The model under review builds one solid part; all positions refer to its coordinate system, in mm. Face numbers are marked on the shaded views. A direction names the side the tool comes from. Coordinates: 2 decimals unless noted, no trailing zeros. Write each loop counter-clockwise with the first axis right and the second up, starting at its lowest first coordinate (ties: lowest second). Pieces come first, ordered by that corner, then holes.
```python
from build123d import *

# Parameters (mm, degrees)
SKETCH1_R               = 20
BOSS_EXTRUDE1_DEPTH     = 60
CUT_EXTRUDE1_DEPTH      = 67.332495807
CUT_EXTRUDE1_DEPTH_BACK = 67.332495807
SKETCH2_R               = 10
FILLET1_R               = 3
SKETCH22_R              = 17
BOSS_EXTRUDE4_DEPTH     = 100
CUT_EXTRUDE4_DEPTH      = 100
CUT_EXTRUDE4_DEPTH_BACK = 100
SKETCH19_R              = 10
CUT_EXTRUDE5_START      = -80
CUT_EXTRUDE5_DEPTH      = 80


with BuildPart() as part:
    # Sketch1 → Boss-Extrude1 (new body)
    with BuildSketch(Plane.XY):
        Circle(SKETCH1_R)
    extrude(amount=BOSS_EXTRUDE1_DEPTH)

    # Sketch2 → Cut-Extrude1 (cut, two sides: drawn at the far end of the back side and taken through both)
    with BuildSketch(Plane(origin=(0, 0, 0), x_dir=(1, 0, 0), z_dir=(0, 1, 0)).offset(-CUT_EXTRUDE1_DEPTH_BACK)):
        with Locations(Location((0, -30, 0), (0, 0, 270))):
            Circle(SKETCH2_R)
    extrude(amount=CUT_EXTRUDE1_DEPTH + CUT_EXTRUDE1_DEPTH_BACK, mode=Mode.SUBTRACT)

    # Fillet1
    fillet1_edges = [part.edges().sort_by_distance(p)[0] for p in [
        (-20, 0, 0),
        (-20, 0, 60),
    ]]
    fillet(fillet1_edges, radius=FILLET1_R)

    # Sketch22 → Boss-Extrude4 (add)
    with BuildSketch(Plane.XY.offset(60)):
        Circle(SKETCH22_R)
    extrude(amount=BOSS_EXTRUDE4_DEPTH)

    # Sketch19 → Cut-Extrude4 (cut, two sides: drawn at the far end of the back side and taken through both)
    with BuildSketch(Plane(origin=(0, 0, 0), x_dir=(1, 0, 0), z_dir=(0, 1, 0)).offset(-CUT_EXTRUDE4_DEPTH_BACK)):
        with Locations(Location((0, -120, 0), (0, 0, 90))):
            Circle(SKETCH19_R)
    extrude(amount=CUT_EXTRUDE4_DEPTH + CUT_EXTRUDE4_DEPTH_BACK, mode=Mode.SUBTRACT)

    # Sketch23 → Cut-Extrude5 (cut)
    with BuildSketch(Plane.XY.offset(160).offset(CUT_EXTRUDE5_START)):
        with BuildLine():
            ThreePointArc((12.56265543, 11.453370183), (0, 17), (-12.56265543, 11.453370183))
            Line((-12.56265543, 11.453370183), (12.56265543, 11.453370183))
        make_face()
        with BuildLine():
            Line((-12.56265543, -11.453370183), (-12.56265543, 11.453370183))
            ThreePointArc((-12.56265543, 11.453370183), (-17, 0), (-12.56265543, -11.453370183))
        make_face()
        with BuildLine():
            Line((12.56265543, -11.453370183), (-12.56265543, -11.453370183))
            ThreePointArc((-12.56265543, -11.453370183), (0, -17), (12.56265543, -11.453370183))
        make_face()
        with BuildLine():
            ThreePointArc((17, 0), (15.851894876, 6.141451689), (12.56265543, 11.453370183))
            Line((12.56265543, 11.453370183), (12.56265543, -11.453370183))
            ThreePointArc((12.56265543, -11.453370183), (15.851894876, -6.141451689), (17, 0))
        make_face()
    extrude(amount=CUT_EXTRUDE5_DEPTH, mode=Mode.SUBTRACT)


solid = part.part
```
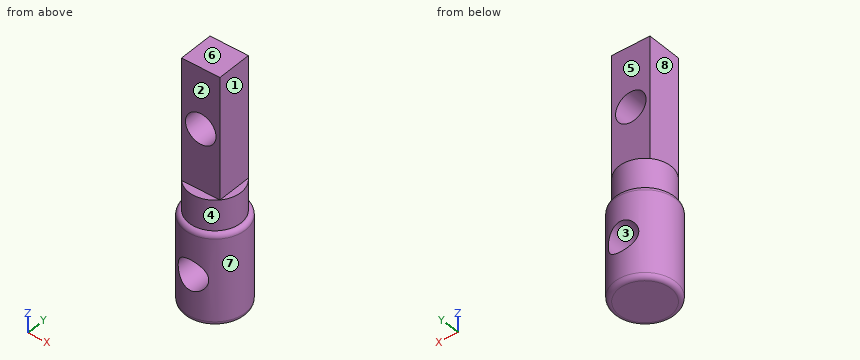
Item 1: Machinability: for the marked faces 4, 5, 6, 7 and 8, which of the approach directions +Z, -Z, +X, -X, +Y, -Y give a long, thin tool a straight path to every point of the face, cutting with its end or side? Answer none if there is none.
Solved:
face 4: +Z
face 5: +Z, +X, -X, +Y
face 6: +Z, +X, -X, +Y, -Y
face 7: +Z, -Z
face 8: +Z, -X, +Y, -Y
Item 2: For pin 1 (6 mm diameter, centred on x = 1, z = 50, fed in from +Y); pin 2 (5 mm diameter, centred on x = 15.5, z = 102.5, fed in from -Y); pin 3 (20 mm diameter, centred on x = -5, z = 116, fed in from -Y); pin 4 (1 mm diameter, centred on x = 1, z = 71, fed in from -Y), all flat-tipped, find the tip position at first contact; note any pin that passes through.
Solved:
pin 1: stops at y = 20
pin 2: passes through
pin 3: stops at y = -11.45
pin 4: stops at y = -16.99
Item 3: Take a section at D-D, the plane z = 138.5. Write out the cut boundary in (x, y).
Solved:
outline: (-12.56, -11.45) - (12.56, -11.45) - (12.56, 11.45) - (-12.56, 11.45) - close
Item 4: To check wall thickness, follow line 1 along X through (y, z) = (-0.5, 30); line 2 along X through (y, z) = (-4, 120); line 3 along Z through (x, y) = (-1, 0). State the ranges of each line that lie inside material, in increasing order.
Solved:
line 1: x = -19.99 to -10, 10 to 19.99
line 2: x = -12.56 to -10, 10 to 12.56
line 3: z = 0 to 20.05, 39.95 to 110.05, 129.95 to 160
Item 5: Take a section at A-A, the plane x = 0. Write out the cut boundary in (y, z).
Solved:
outline: (-20, 3) arc R3 ccw to (-17, 0) - (17, 0) arc R3 ccw to (20, 3) - (20, 20) - (-20, 20) - close; (-20, 40) - (20, 40) - (20, 57) arc R3 ccw to (17, 60) - (17, 80) - (11.45, 80) - (11.45, 110) - (-11.45, 110) - (-11.45, 80) - (-17, 80) - (-17, 60) arc R3 ccw to (-20, 57) - close; (-11.45, 130) - (11.45, 130) - (11.45, 160) - (-11.45, 160) - close
Item 6: Mouldability with a two-part tool opening along X and no side actions: class the marked faces 1, 2 and 3 as pulls with the +X half, pulls with the -X half, needs draft (parallel to the pull), parting line crosses it, or undercut.
Solved:
face 1: pulls with the +X half
face 2: needs draft
face 3: undercut
Item 7: Take a section at C-C, the plane z = 36. Write out the cut boundary in (x, y).
Solved:
outline: (-8, -18.33) - (-8, 18.33) arc R20 ccw to start; (8, -18.33) arc R20 ccw to (8, 18.33) - close
Item 8: Take a section at B-B, the plane y = 0. Write out the cut boundary in (x, z), plus the area to 3 significant figures.
Solved:
outline: (-20, 3) arc R3 ccw to (-17, 0) - (17, 0) arc R3 ccw to (20, 3) - (20, 57) arc R3 ccw to (17, 60) - (17, 80) - (12.56, 80) - (12.56, 160) - (-12.56, 160) - (-12.56, 80) - (-17, 80) - (-17, 60) arc R3 ccw to (-20, 57) - close; hole circle Ø20 at (0, 30); hole circle Ø20 at (0, 120)
area: 4,450 mm2
